Can you work these out from the model? Positions are in its coordinate system, mm. Face numbers are marked on the shaded views. A direction names the side the tool comes from. Round coordinates to 2 decimals unless told otherwise and drop trailing zeros. Order: outer loops, then holes, each group sorted by start corner. A loop starts at its lowest first (then second) coordinate and runs counter-clockwise, first axis right, second up. Notation, with made-up numbers: (55.25, 24.25) -> (101.25, 24.25) arc R18 cw to (101.25, 43.25) -> close; hole circle Ø2 at (29, 24). An arc over 180 degrees is marked (long way). One line per item, written item: value.
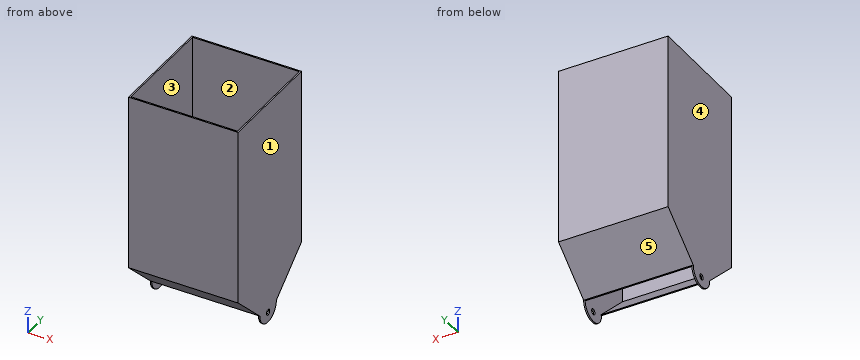
```python
from build123d import *

# Parameters (mm, degrees)
SKETCH1_W               = 154
SKETCH1_H               = 154
SKETCH1_W_2             = 150
SKETCH1_H_2             = 150
BOSS_EXTRUDE1_DEPTH     = 250
BOSS_EXTRUDE6_DEPTH     = 2
BOSS_EXTRUDE7_START     = -152
BOSS_EXTRUDE7_DEPTH     = 2
CUT_EXTRUDE1_DEPTH      = 304.553949235
CUT_EXTRUDE1_DEPTH_BACK = 304.553949235
SKETCH8_R               = 4


with BuildPart() as part:
    # Sketch1 → Boss-Extrude1 (new body)
    with BuildSketch(Plane.XY):
        Rectangle(SKETCH1_W, SKETCH1_H)
        Rectangle(SKETCH1_W_2, SKETCH1_H_2, mode=Mode.SUBTRACT)
    extrude(amount=BOSS_EXTRUDE1_DEPTH)

    # Sketch3 → Loft1 section 0
    with BuildSketch(Plane.XY.offset(-50)):
        with BuildLine():
            Line((-77, 15.887313735), (77, 15.887313735))
            Line((77, 15.887313735), (77, -24.112686265))
            Line((77, -24.112686265), (-77, -24.112686265))
            Line((-77, -24.112686265), (-77, 15.887313735))
        make_face()
    # Sketch2 → Loft1 section 1
    with BuildSketch(Plane(origin=(0, 0, 0), x_dir=(-1, 0, 0), z_dir=(0, 0, -1))):
        with BuildLine():
            Line((-77, 77), (77, 77))
            Line((77, 77), (77, -77))
            Line((77, -77), (-77, -77))
            Line((-77, -77), (-77, 77))
        make_face()
    loft()

    # Sketch3<3> → Cut-Loft1 section 0
    with BuildSketch(Plane.XY.offset(-50)):
        with BuildLine():
            Line((-75, 13.887313735), (-75, -22.112686265))
            Line((-75, -22.112686265), (75, -22.112686265))
            Line((75, -22.112686265), (75, 13.887313735))
            Line((75, 13.887313735), (-75, 13.887313735))
        make_face()
    # Sketch1<2> → Cut-Loft1 section 1
    with BuildSketch(Plane.XY):
        with BuildLine():
            Line((-75, 75), (75, 75))
            Line((75, 75), (75, -75))
            Line((75, -75), (-75, -75))
            Line((-75, -75), (-75, 75))
        make_face()
    loft(mode=Mode.SUBTRACT)

    # Sketch7 → Boss-Extrude6 (add)
    with BuildSketch(Plane(origin=(77, 0, 0), x_dir=(0, 0, -1), z_dir=(1, 0, 0))):
        with BuildLine():
            Line((50, 15.887313735), (50, -24.112686265))
            ThreePointArc((50, -24.112686265), (70, -4.112686265), (50, 15.887313735))
        make_face()
    extrude(amount=-BOSS_EXTRUDE6_DEPTH)

    # Sketch7<2> → Boss-Extrude7 (add)
    with BuildSketch(Plane(origin=(77, 0, 0), x_dir=(0, 0, -1), z_dir=(1, 0, 0)).offset(BOSS_EXTRUDE7_START)):
        with BuildLine():
            Line((50, 15.887313735), (50, -24.112686265))
            ThreePointArc((50, -24.112686265), (70, -4.112686265), (50, 15.887313735))
        make_face()
    extrude(amount=-BOSS_EXTRUDE7_DEPTH)

    # Sketch8 → Cut-Extrude1 (cut, two sides: drawn at the far end of the back side and taken through both)
    with BuildSketch(Plane(origin=(77, 0, 0), x_dir=(0, 0, -1), z_dir=(1, 0, 0)).offset(-CUT_EXTRUDE1_DEPTH_BACK)):
        with Locations(Location((55.834353072, -4.112686265, 0), (0, 0, 90))):
            Circle(SKETCH8_R)
    extrude(amount=CUT_EXTRUDE1_DEPTH + CUT_EXTRUDE1_DEPTH_BACK, mode=Mode.SUBTRACT)


solid = part.part
```
Q1. We'd pull the mould along X, two halves only. Please class the marked faces 3, 4 and 5: released by +X, released by -X, zero draft, split by the parting line, or undercut.
Answers below:
face 3: undercut
face 4: released by -X
face 5: zero draft
Q2. On a 3-axis mill with a long thin cutter (end or side, diameter ignored), from which of +Z, -Z, +X, -X, +Y, -Y can I reach the whole of each face in a straight line? I mean the marked faces 1 and 2. Say none if no direction works.
Answers below:
face 1: +Z, -Z, +X, +Y, -Y
face 2: +Z
Q3. I want a section at A-A on x = 34.5. List the corners of the cut face in (y, z) for me.
Answers below:
outline: (-77, 0) -> (-24.11, -50) -> (-22.11, -50) -> (-75, 0) -> (-75, 250) -> (-77, 250) -> close; (13.89, -50) -> (15.89, -50) -> (77, 0) -> (77, 250) -> (75, 250) -> (75, 0) -> close
Q4. Please list where these lines run through material, in increasing order: line 1 along X through (y, z) = (-35.5, 6); line 2 along Y through (x, z) = (50, -26.5).
Answers below:
line 1: -77 to -75, 75 to 77
line 2: -48.97 to -46.97, 42.61 to 44.61
Q5. I want a section at C-C on y = -50. List the corners of the cut face in (x, z) for me, plus the area to 3 significant figures.
Answers below:
outline: (-77, -25.53) -> (77, -25.53) -> (77, 250) -> (75, 250) -> (75, -23.64) -> (-75, -23.64) -> (-75, 250) -> (-77, 250) -> close
area: 1,390 mm^2
Q6. I want a section at B-B on z = 82.5. List the corners of the cut face in (x, y) for me, plus the area to 3 significant figures.
Answers below:
outline: (-77, -77) -> (77, -77) -> (77, 77) -> (-77, 77) -> close; hole (-75, -75) -> (75, -75) -> (75, 75) -> (-75, 75) -> close
area: 1,220 mm^2
Q7. Will these pins go through, and if not, where does the flat tip stop? pin 1 Ø1.6 at (x, y) = (26.5, -23.5) entering from -Z; pin 2 Ø13 at (y, z) = (-4.11, -55.83) entering from -X; pin 3 Ø1 at (x, y) = (-17.5, 27.5) entering from -Z.
Answers below:
pin 1: z = -50
pin 2: x = -77
pin 3: z = -40.91
Q8. I want a section at D-D on y = 41. List the corners of the cut face in (x, z) for me.
Answers below:
outline: (-77, -29.45) -> (77, -29.45) -> (77, 250) -> (75, 250) -> (75, -27.82) -> (-75, -27.82) -> (-75, 250) -> (-77, 250) -> close
